Autodesk Fusion 360 part; units mm, degrees
sketch "Sketch1" plane through (0, 0, 0) normal (0, 0, 1) x (1, 0, 0)
  circle A0 centre (0, 0) radius 19
  circle A1 centre (0, 0) radius 16
  dimension "d6" = 38
  dimension "d7" = 32
extrude "Extrude1" add sketch "Sketch1" along normal blind 119
sketch "Sketch2" plane through (0, 0, 0) normal (0, 0, 1) x (1, 0, 0)
  line L0 (32, 6) -> (-32, 6)
  line L1 (-32, 6) -> (-32, -6)
  line L2 (-32, -6) -> (32, -6)
  line L3 (32, -6) -> (32, 6)
  line L4 (32, 6) -> (-32, -6) construction
  line L5 (-32, 6) -> (32, -6) construction
  dimension "d10" = 64
  dimension "d11" = 12
extrude "Extrude2" cut sketch "Sketch2" along normal blind 31
ref_plane "WorkPlane1" through (0, 0, 119) normal (0, 0, 1) x (1, 0, 0)
sketch "Sketch3" plane through (0, 0, 119) normal (0, 0, 1) x (1, 0, 0)
  line L0 (32, 6) -> (-32, 6)
  line L1 (-32, 6) -> (-32, -6)
  line L2 (-32, -6) -> (32, -6)
  line L3 (32, -6) -> (32, 6)
  line L4 (32, 6) -> (-32, -6) construction
  line L5 (-32, 6) -> (32, -6) construction
  dimension "d15" = 64
  dimension "d16" = 12
extrude "Extrude3" cut sketch "Sketch3" against normal blind 66
equation "discDia = 32 mm"
equation "discHeight = 11 mm"
equation "gutterRim = 12 mm"
equation "gutterDepth = 31 mm"
equation "wall = 3 mm"
equation "d6 = discDia + wall * 2"
equation "d7 = discDia"
equation "d8 = gutterDepth + discAreaHeight"
equation "d10 = discDia * 2"
equation "d11 = gutterRim"
equation "d12 = gutterDepth"
equation "d14 = gutterDepth + discAreaHeight"
equation "d15 = discDia * 2"
equation "d16 = gutterRim"
equation "d17 = -discAreaHeight + 2 * discHeight"
equation "discAreaHeight = discHeight * 8"
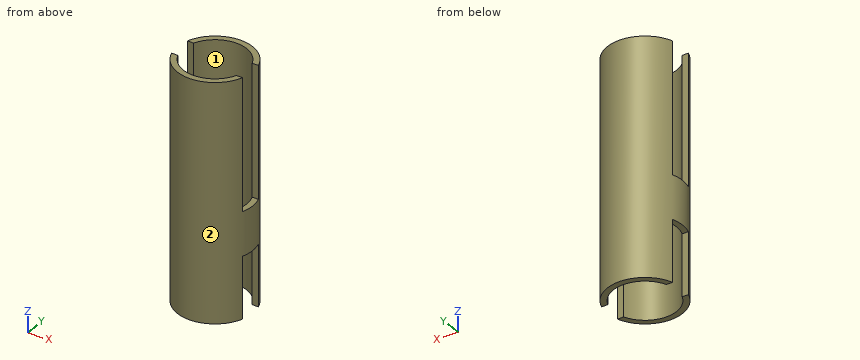
Input: part model. Units: mm. Frame: model coordinates. Face numbers are marked on the shaded views. Round coordinates to 2 decimals unless told otherwise and drop trailing zeros. Loops run counter-clockwise (first coordinate to the right, second up) from the corner with the lowest first, then second, coordinate; pieces in that order, holes last. Notation, with made-up numbers: (60.5, 54) -> (66.5, 54) arc R24 cw to (66.5, 69) -> close; hole circle Ø5 at (11.5, 1). An arc over 180 degrees is marked (long way). Use one line per item in the form item = value. Start each with the question number.
Item 1: Section query A-A on z = 75. Return the cut outline in (x, y), then the cut area to 3 significant figures.
Item 2: Contact query for flat-ended pins moving along their axis: pin 1 Ø1.3 at (x, y) = (-17, -1.5) entering from -Z; pin 2 Ø5 at (y, z) = (-6.5, 90) entering from +X; pin 3 Ø3.5 at (x, z) = (-16, 21.5) entering from -Y. Output: stop coordinate, or through.
Item 3: Material intervals for L1, parallel to X at y = -6, z = 45.5; L2, parallel to X at y = 0, z = 37.5; L3, parallel to Y at x = 11.5, z = 12.5, sorted ascending. Write a range as from..to.
Item 4: Mould query, pull axis X, two halves, no side actions, for the marked faces 1 and 2. Classes: pulls with the +X half, pulls with the -X half, needs draft (parallel to the pull), parting line crosses it, or undercut.
Item 5: Section query B-B on x = 0. Return the cut outline in (y, z).
Item 6: Section query C-C on z = 35. Return the cut outline in (x, y), then the cut area to 3 significant figures.
Ans:
q1.outline = (-18.03, -6) arc R19 ccw to (18.03, -6) -> (14.83, -6) arc R16 cw to (-14.83, -6) -> close; (-18.03, 6) -> (-14.83, 6) arc R16 cw to (14.83, 6) -> (18.03, 6) arc R19 ccw to start
q1.area = 256 mm^2
q2.pin_1 = 31
q2.pin_2 = 18.03
q2.pin_3 = -12.57
q3.L1 = -18.03..-14.83, 14.83..18.03
q3.L2 = -19..-16, 16..19
q3.L3 = -15.12..-11.12, 11.12..15.12
q4.face_1 = undercut
q4.face_2 = parting line crosses it
q5.outline = (-19, 0) -> (-16, 0) -> (-16, 119) -> (-19, 119) -> close; (16, 0) -> (19, 0) -> (19, 119) -> (16, 119) -> close
q6.outline = circle Ø38 at (0, 0); hole circle Ø32 at (0, 0)
q6.area = 330 mm^2
